Check sheet for the modelled part. Datum: model origin and axes. Units: mm. A direction names the side the tool comes from. Give positions to 0.01 mm unless a question says otherwise; leave off trailing zeros. Loops run counter-clockwise (first coordinate to the right, second up) from the corner with the lowest first, then second, coordinate; pieces in that order, holes last. Notation, with made-up numbers: (85, 76) - (92, 76) arc R26 cw to (92, 114) - close; hole circle Ø2 at (-40, -35.75). An arc over 180 degrees is marked (long way). Use one line per item in the form item = value.
Autodesk Inventor part; units mm, degrees
ref_plane "YZ Plane" through (0, 0, 0) normal (1, 0, 0) x (0, 1, 0)
ref_plane "XZ Plane" through (0, 0, 0) normal (0, 1, 0) x (-1, 0, 0)
ref_plane "XY Plane" through (0, 0, 0) normal (0, 0, 1) x (1, 0, 0)
sketch "Sketch1" plane through (0, 0, 0) normal (0, 1, 0) x (-1, 0, 0)
  line L0 (13.0479, 11.7432) -> (-12.3521, 11.7432)
  line L1 (-12.3521, 11.7432) -> (-12.3521, -13.6568)
  line L2 (-12.3521, -13.6568) -> (13.0479, -13.6568)
  line L3 (13.0479, -13.6568) -> (13.0479, 11.7432)
  point P0 (0, 0)
  dimension "d0" = 25.4
  dimension "d1" = 25.4
extrude "Extrusion1" add sketch "Sketch1" along normal blind 25.4
sketch "Sketch2" plane through (-13.0479, 0, 11.7432) normal (0, 0, 1) x (1, 0, 0)
  line L0 (2.8121, 3.3867) -> (20.955, 3.3867)
  line L1 (20.955, 3.3867) -> (20.955, 20.5619)
  line L2 (20.955, 20.5619) -> (2.8121, 20.5619)
  line L3 (2.8121, 20.5619) -> (2.8121, 3.3867)
  point P0 (13.0479, 0)
extrude "Extrusion2" cut sketch "Sketch2" against normal blind 25.4
properties part number "Zohair did a thing"
Item 1: Gauge pin test, flat end, axial feed: P1, Ø6, axis at x = -4.5, y = 4, coming from the +Z side. Record the tip position at first contact, or that the pin passes through.
Answer block:
P1 = 11.74
Item 2: Section check A-A on x = -4. Record the boundary of the cut face in (y, z), then the cut area to 3 significant figures.
Answer block:
outline = (0, -13.66) - (3.39, -13.66) - (3.39, 11.74) - (0, 11.74) - close; (20.56, -13.66) - (25.4, -13.66) - (25.4, 11.74) - (20.56, 11.74) - close
area = 209 mm2
Item 3: Access from +Z, -Z, +X, -X, +Y, -Y to the whole of each face (thin tool, end or side, straight path). Record for faces 4 (the face through (-1, 20.562, -1)), 5 (the face through (0, 0, -1)).
Answer block:
face_4 = +Z, -Z
face_5 = +Z, -Z, +X, -X, -Y
Item 4: Thickness scan on L1, parallel to Y at x = -9.75, z = -2.5; L2, parallel to X at y = 3.5, z = 10. Record the ranges inside material, lowest first.
Answer block:
L1 = 0 to 3.39, 20.56 to 25.4
L2 = -13.05 to -10.24, 7.91 to 12.35
Item 5: Section check B-B on z = -8.25. Record the boundary of the cut face in (x, y).
Answer block:
outline = (-13.05, 0) - (12.35, 0) - (12.35, 25.4) - (-13.05, 25.4) - close; hole (-10.24, 3.39) - (7.91, 3.39) - (7.91, 20.56) - (-10.24, 20.56) - close
Item 6: Section check C-C on y = 13.25. Record the boundary of the cut face in (x, z), then the cut area to 3 significant figures.
Answer block:
outline = (-13.05, -13.66) - (-10.24, -13.66) - (-10.24, 11.74) - (-13.05, 11.74) - close; (7.91, -13.66) - (12.35, -13.66) - (12.35, 11.74) - (7.91, 11.74) - close
area = 184 mm2
Item 7: Mould release check, pull along Y, two halves, no side actions. Record for faces 1 (the face through (12.352, 13, -1)), 2 (the face through (0, 25.4, -1)), 3 (the face through (-10.236, 12, -1)): released by +Y, released by -Y, zero draft, split by the parting line, or undercut.
Answer block:
face_1 = zero draft
face_2 = released by +Y
face_3 = undercut
